Here's how the part is built. I have some questions about the finished solid (model axes, mm). Round coordinates to 2 decimals unless told otherwise and drop trailing zeros. Write each loop counter-clockwise with the first axis right and the second up, starting at its lowest first coordinate (ties: lowest second). Pieces come first, ordered by that corner, then holes. Notation, with made-up numbers: (80, 87.25) -> (138, 87.25) arc R30 cw to (138, 122.25) -> close; hole circle Ø1 at (-5, -40). An arc over 180 degrees is marked (long way). Put each result on its own line as item: value. Start each with the question number.
1) I want a section at A-A, the plane y = -8. List the corners of the cut face in (x, z) for me.
2) I want a section at D-D, the plane x = 55.5. List the corners of the cut face in (y, z) for me.
3) Will these pins go through, and if not, where does the flat tip stop? P1, Ø0.9, axis at x = 4.5, z = 1.5, coming from the +Y side; P2, Ø3, axis at x = 25, y = 0, coming from the +Z side; P3, Ø0.7, axis at x = 48, z = 2, coming from the +Y side; P4, Ø0.9, axis at x = 5, z = 2, coming from the +Y side.
4) I want a section at C-C, the plane y = 5. List the corners of the cut face in (x, z) for me, then the cut area to 3 significant figures.
5) I want a section at B-B, the plane x = 4. List the corners of the cut face in (y, z) for me, then the cut area to 3 significant figures.
6) If I drill on line 1 along X through (y, z) = (-24, 2.9); line 2 along X through (y, z) = (-9.5, 2.7); line 3 along X through (y, z) = (11, 1.6), over which ranges is the centre line in solid material (lowest first)? Write a range as [from, to].
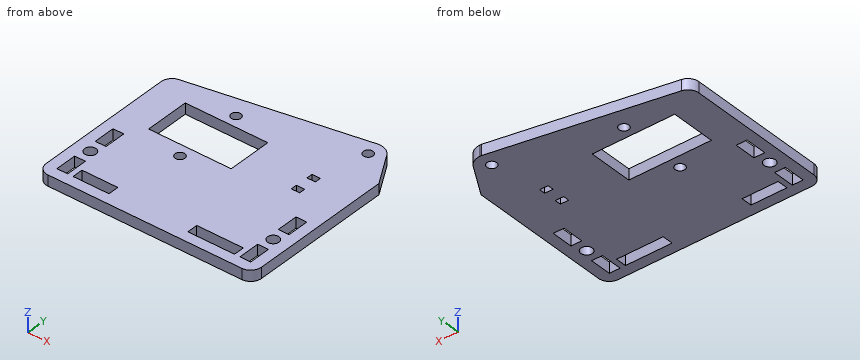
from build123d import *

# Parameters (mm, degrees)
SKETCH_1_R          = 1.359
SKETCH_1_W          = 3
SKETCH_1_H          = 6.001
SKETCH_1_W_2        = 10
SKETCH_1_H_2        = 3
SKETCH_1_W_3        = 12.999
SKETCH_1_W_4        = 2.329
SKETCH_1_H_3        = 1.693
SKETCH_1_W_5        = 23
SKETCH_1_H_4        = 12.399
EXTRUDE_1_DEPTH     = 3
SKETCH_2_R          = 1.6
CUT_EXTRUDE_1_DEPTH = 67.26469212


with BuildPart() as part:
    # 草图1 → 凸台-拉伸1 (new body)
    with BuildSketch(Plane(origin=(0, 0, 0), x_dir=(-1, 0, 0), z_dir=(0, 0, -1))):
        with BuildLine():
            Line((-57, -27.964431369), (-3, -27.964431369))
            ThreePointArc((-3, -27.964431369), (-0.878679656, -27.085751712), (0, -24.964431369))
            Line((0, -24.964431369), (0, 14.035588089))
            ThreePointArc((0, 14.035588089), (-0.693884476, 15.954397926), (-2.454554127, 16.985586191))
            Line((-2.454554127, 16.985586191), (-50.782638999, 25.921305316))
            Line((-50.782638999, 25.921305316), (-51.262778196, 25.921305316))
            ThreePointArc((-51.262778196, 25.921305316), (-53.258114674, 25.388095235), (-54.721484389, 23.930621486))
            Line((-54.721484389, 23.930621486), (-60, 14.844527968))
            Line((-60, 14.844527968), (-60, -24.964431369))
            ThreePointArc((-60, -24.964431369), (-59.121320344, -27.085751712), (-57, -27.964431369))
        make_face()
        with Locations(Location((-55.5, -15.464331369, 0), (0, 0, 180))):
            Circle(SKETCH_1_R, mode=Mode.SUBTRACT)
        with Locations(Location((-4.5, -15.464331369, 0), (0, 0, 180))):
            Circle(SKETCH_1_R, mode=Mode.SUBTRACT)
        with Locations(Location((-20.499, -4.535331369, 0), (0, 0, 180))):
            Circle(SKETCH_1_R, mode=Mode.SUBTRACT)
        with Locations(Location((-20.499, 14.465668631, 0), (0, 0, 180))):
            Circle(SKETCH_1_R, mode=Mode.SUBTRACT)
        with Locations(Location((-51.251, 21.869668631, 0), (0, 0, 180))):
            Circle(SKETCH_1_R, mode=Mode.SUBTRACT)
        with Locations((-4.501, -8.964831369)):
            Rectangle(SKETCH_1_W, SKETCH_1_H, mode=Mode.SUBTRACT)
        with Locations((-4.501, -21.963831369)):
            Rectangle(SKETCH_1_W, SKETCH_1_H, mode=Mode.SUBTRACT)
        with Locations((-55.5, -21.963831369)):
            Rectangle(SKETCH_1_W, SKETCH_1_H, mode=Mode.SUBTRACT)
        with Locations((-55.5, -8.964831369)):
            Rectangle(SKETCH_1_W, SKETCH_1_H, mode=Mode.SUBTRACT)
        with Locations((-12.5, -23.464331369)):
            Rectangle(SKETCH_1_W_2, SKETCH_1_H_2, mode=Mode.SUBTRACT)
        with Locations((-45.9995, -23.464331369)):
            Rectangle(SKETCH_1_W_3, SKETCH_1_H_2, mode=Mode.SUBTRACT)
        with Locations((-47.8955, 7.444168631)):
            Rectangle(SKETCH_1_W_4, SKETCH_1_H_3, mode=Mode.SUBTRACT)
        with Locations((-47.8435, 2.205168631)):
            Rectangle(SKETCH_1_W_4, SKETCH_1_H_3, mode=Mode.SUBTRACT)
        with Locations((-20.5, 5.035168631)):
            Rectangle(SKETCH_1_W_5, SKETCH_1_H_4, mode=Mode.SUBTRACT)
    extrude(amount=-EXTRUDE_1_DEPTH)

    # 草图2 → 切除-拉伸1 (cut, through all)
    with BuildSketch(Plane.XY.offset(3)):
        with Locations((55.5, -15.464331369)):
            Circle(SKETCH_2_R)
        with Locations((4.5, -15.464331369)):
            Circle(SKETCH_2_R)
    extrude(amount=-CUT_EXTRUDE_1_DEPTH, mode=Mode.SUBTRACT)


solid = part.part
Findings:
1. outline: (0, 0) -> (3, 0) -> (3, 3) -> (0, 3) -> close; (6, 0) -> (54, 0) -> (54, 3) -> (6, 3) -> close; (57, 0) -> (60, 0) -> (60, 3) -> (57, 3) -> close
2. outline: (-27.96, 0) -> (-24.96, 0) -> (-24.96, 3) -> (-27.96, 3) -> close; (-18.96, 0) -> (-17.06, 0) -> (-17.06, 3) -> (-18.96, 3) -> close; (-13.86, 0) -> (-11.97, 0) -> (-11.97, 3) -> (-13.86, 3) -> close; (-5.96, 0) -> (22.59, 0) -> (22.59, 3) -> (-5.96, 3) -> close
3. P1: stops at y = 17.45
3. P2: stops at z = 3
3. P3: stops at y = 25.47
3. P4: stops at y = 17.54
4. outline: (0, 0) -> (9, 0) -> (9, 3) -> (0, 3) -> close; (32, 0) -> (60, 0) -> (60, 3) -> (32, 3) -> close
4. area: 111 mm2
5. outline: (-27.96, 0) -> (-24.96, 0) -> (-24.96, 3) -> (-27.96, 3) -> close; (-18.96, 0) -> (-16.98, 0) -> (-16.98, 3) -> (-18.96, 3) -> close; (-13.94, 0) -> (-11.97, 0) -> (-11.97, 3) -> (-13.94, 3) -> close; (-5.96, 0) -> (17.27, 0) -> (17.27, 3) -> (-5.96, 3) -> close
5. area: 90.6 mm2
6. line 1: x = [0, 3], [6, 7.5], [17.5, 39.5], [52.5, 54], [57, 60]
6. line 2: x = [0, 3], [6, 54], [57, 60]
6. line 3: x = [0, 9], [32, 60]
